Study the drawing (mm; zero at the part's minimum x, y, z) and answer. A direction names the side the tool comes from. Round coordinates to 2 decimals unless told otherwise and drop trailing zeros. Order: outer loops, then holes, each group sorted by start corner. A loop starts at its lowest first (then second) coordinate and runs counter-clockwise, first axis right, second up. Notation, with made-up numbers: (-5.75, 69.25) - (38.25, 69.25) arc R12 cw to (38.25, 80.25) - close; hole circle Ø8 at (-4, -31). An arc over 180 degrees is marked (long way). Put each result on its own line as item: value. Start each with the question number.
Q1. For a pull along Y with two mould halves and no side action, classify the marked faces 1, 2 and 3 as pulls with the +Y half, pulls with the -Y half, needs draft (parallel to the pull), parting line crosses it, or undercut.
Q2. Section D-D on x = 2 is taken. Give the vertices of the cut face in (y, z).
Q3. Section B-B on x = 10 is taken. Give the vertices of the cut face in (y, z), then the cut area to 3 significant figures.
Q4. Each of these flat-tipped pins is pushed along its axis until it touches: pin 1 Ø8.5 at (x, z) = (11.5, 8.5) entering from -Y; pin 2 Ø3 at (y, z) = (5, 5) entering from +X; pin 3 Ø8 at (y, z) = (5, 4) entering from +X. Where does it stop, or does it pass through?
Q5. Which of the six approach directions +Z, -Z, +X, -X, +Y, -Y give full straight-line access (tool end or side, diameter ignored) to the marked faces 4 and 5?
Q6. Section C-C on y = 3.5 is taken. Give the vertices of the cut face in (x, z).
Q7. Section A-A on z = 15 is taken. Give the vertices of the cut face in (x, y).
Q8. Find the intervals of material crossed by line 1 along Y through (x, z) = (2.3, 15); line 2 along X through (y, z) = (12.9, 10); line 3 along Z through (x, y) = (2.75, 5.5), in increasing order. Write a range as from..to.
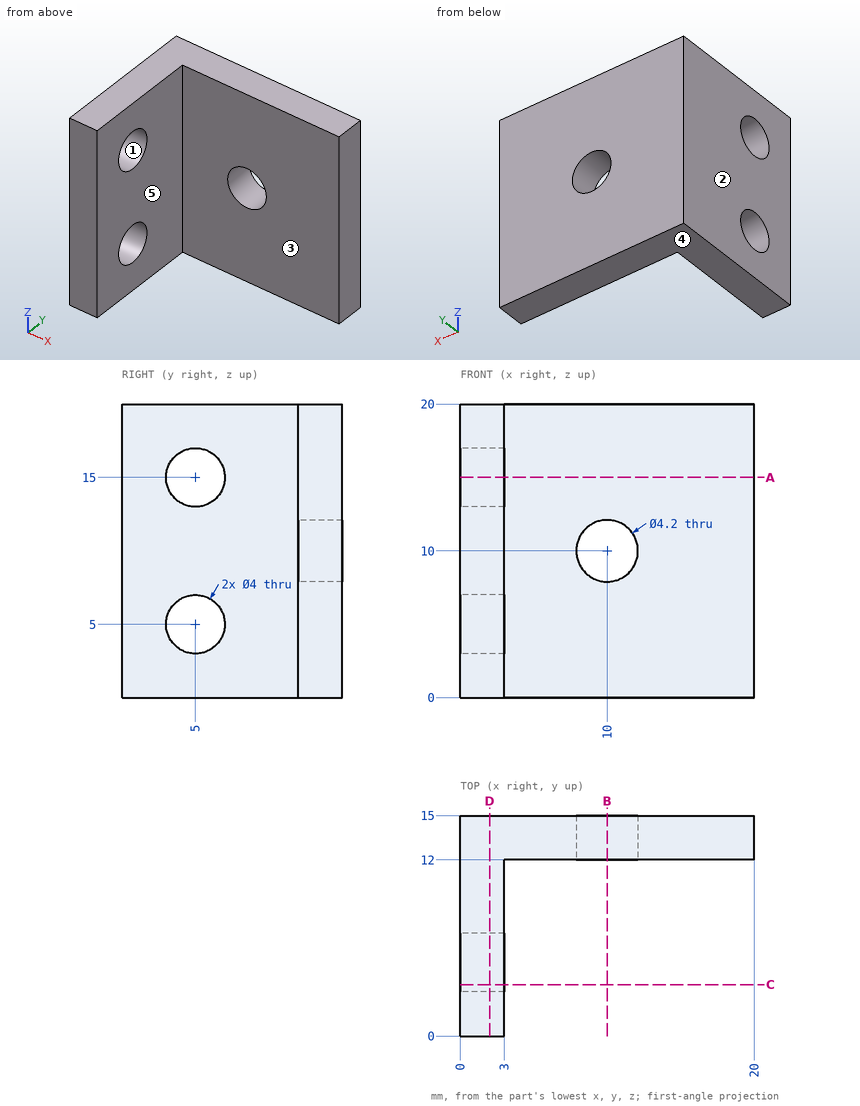
Findings:
1. face 1: undercut
1. face 2: needs draft
1. face 3: pulls with the -Y half
2. outline: (0, 0) - (15, 0) - (15, 20) - (0, 20) - close; hole circle Ø4 at (5, 5); hole circle Ø4 at (5, 15)
3. outline: (12, 0) - (15, 0) - (15, 7.9) - (12, 7.9) - close; (12, 12.1) - (15, 12.1) - (15, 20) - (12, 20) - close
3. area: 47.4 mm2
4. pin 1: y = 12
4. pin 2: through
4. pin 3: x = 3
5. face 4: -Z, +X, -X, +Y, -Y
5. face 5: +Z, -Z, +X, -Y
6. outline: (0, 0) - (3, 0) - (3, 3.68) - (0, 3.68) - close; (0, 6.32) - (3, 6.32) - (3, 13.68) - (0, 13.68) - close; (0, 16.32) - (3, 16.32) - (3, 20) - (0, 20) - close
7. outline: (0, 0) - (3, 0) - (3, 3) - (0, 3) - close; (0, 7) - (3, 7) - (3, 12) - (20, 12) - (20, 15) - (0, 15) - close
8. line 1: 0..3, 7..15
8. line 2: 0..7.9, 12.1..20
8. line 3: 0..3.06, 6.94..13.06, 16.94..20
